The model under review builds one solid part; all positions refer to its coordinate system, in mm. Face numbers are marked on the shaded views. A direction names the side the tool comes from. Give positions to 0.01 mm unless a question says otherwise; leave off trailing zeros. Loops run counter-clockwise (first coordinate to the right, second up) from the corner with the lowest first, then second, coordinate; pieces in that order, holes last. Notation, with made-up numbers: (80, -26.75) - (116, -26.75) arc R10 cw to (116, -21.75) - close; hole circle Ø5 at (58, -20). An arc over 180 degrees is marked (long way). Answer as a JSON object with one key per item and string values.
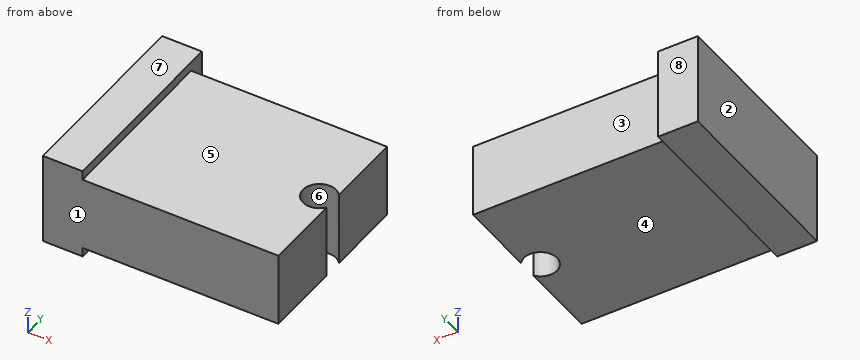
from build123d import *

# Parameters (mm, degrees)
F1_DEPTH = 5.6
F2_D     = 2.5
F2_DEPTH = 12
F3_W     = 13.2
F3_H     = 5.6
F4_DEPTH = 3


with BuildPart() as f1:
    # F0 (on Top) → F1 (new body)
    with BuildSketch(Plane.XY):
        with BuildLine():
            Line((7.4, 6.6), (-7.4, 6.6))
            Line((-7.4, 6.6), (-7.4, 0))
            Line((-7.4, 0), (5.3, 0))
            ThreePointArc((5.3, 0), (6.165479, 1.074709), (7.4, 0.458258))
            Line((7.4, 0.458258), (7.4, 6.6))
        make_face()
        with BuildLine():
            Line((5.3, 0), (-7.4, 0))
            Line((-7.4, 0), (-7.4, -6.6))
            Line((-7.4, -6.6), (7.4, -6.6))
            Line((7.4, -6.6), (7.4, -0.458258))
            ThreePointArc((7.4, -0.458258), (6.165479, -1.074709), (5.3, 0))
        make_face()
        with BuildLine():
            ThreePointArc((7.5, 0), (7.474709, 0.234521), (7.4, 0.458258))
            Line((7.4, 0.458258), (7.4, -0.458258))
            ThreePointArc((7.4, -0.458258), (7.474709, -0.234521), (7.5, 0))
        make_face()
        with BuildLine():
            Line((7.4, -0.458258), (7.4, 0.458258))
            ThreePointArc((7.4, 0.458258), (6.165479, 1.074709), (5.3, 0))
            ThreePointArc((5.3, 0), (6.165479, -1.074709), (7.4, -0.458258))
        make_face()
    extrude(amount=F1_DEPTH)

    # F2
    with Locations(Plane(origin=(0, 0, 0), x_dir=(1, 0, 0), z_dir=(0, 0, -1))):
        with Locations((6.4, 0)):
            Hole(F2_D / 2, depth=F2_DEPTH)

    # F3 (on face) → F4 (join)
    with BuildSketch(Plane(origin=(-7.4, 0, 0), x_dir=(0, -1, 0), z_dir=(-1, 0, 0))):
        Polygon((6.6, 6.3), (-7.9, 6.3), (-7.9, -0.7), (6.6, -0.7), (6.6, 0), (-6.6, 0), (-6.6, 5.6), (6.6, 5.6), align=None)
        with Locations((0, 2.8)):
            Rectangle(F3_W, F3_H)
    extrude(amount=F4_DEPTH)


solid = f1.part
Q1. The part is to be moulded in two halves that separate along Y. For the marked faces 6, 7 and 8, say which applies: +Y half, -Y half, draft (parallel to the pull), parting line (faces both ways), or undercut.
Results:
{"face 6": "undercut", "face 7": "draft", "face 8": "+Y half"}
Q2. Clearance check with flat-ended pins moving along their axes: pin 1 Ø1.5 at (x, z) = (0, 3.5) entering from +Y; pin 2 Ø6 at (x, y) = (-1, -2) entering from -Z. State where each tip first meets the part, or that it passes through.
Results:
{"pin 1": "stops at y = 6.6", "pin 2": "stops at z = 0"}
Q3. Consider section C-C, the plane z = 1. State the section outline as (x, y) points, plus the area to 3 significant figures.
Results:
{"outline": "(-10.4, -6.6) - (7.4, -6.6) - (7.4, -0.75) arc R1.25 cw (long way) to (7.4, 0.75) - (7.4, 6.6) - (-7.4, 6.6) - (-7.4, 7.9) - (-10.4, 7.9) - close", "area": "234 mm^2"}
Q4. Consider section B-B, the plane x = 6.4. State the section outline as (y, z) points.
Results:
{"outline": "(-6.6, 0) - (-1.25, 0) - (-1.25, 5.6) - (-6.6, 5.6) - close; (1.25, 0) - (6.6, 0) - (6.6, 5.6) - (1.25, 5.6) - close"}
Q5. To check wall thickness, follow probe 1 along Y at (x, z) = (6.5, 4); probe 2 along Z at (x, y) = (-1, -4.5); probe 3 along X at (y, z) = (0, 2.45). State the ranges of each line that lie inside material, in increasing order. Write a range as [from, to].
Results:
{"probe 1": "y = [-6.6, -1.25], [1.25, 6.6]", "probe 2": "z = [0, 5.6]", "probe 3": "x = [-10.4, 5.15]"}
Q6. Consider section A-A, the plane y = 1. State the section outline as (x, z) points, plus the area to 3 significant figures.
Results:
{"outline": "(-10.4, -0.7) - (-7.4, -0.7) - (-7.4, 0) - (5.65, 0) - (5.65, 5.6) - (-7.4, 5.6) - (-7.4, 6.3) - (-10.4, 6.3) - close; (7.15, 0) - (7.4, 0) - (7.4, 5.6) - (7.15, 5.6) - close", "area": "95.5 mm^2"}
Q7. Consider section D-D, the plane y = 5.5. State the section outline as (x, z) points, plus the area to 3 significant figures.
Results:
{"outline": "(-10.4, -0.7) - (-7.4, -0.7) - (-7.4, 0) - (7.4, 0) - (7.4, 5.6) - (-7.4, 5.6) - (-7.4, 6.3) - (-10.4, 6.3) - close", "area": "104 mm^2"}
Q8. For the marked faces 1, 2, 3, 4 and 5, list the 3-axis set-ups (+Z, -Z, +X, -X, +Y, -Y) from which the entire face can be reached by the end or side of a thin tool; tool diameter is ignored.
Results:
{"face 1": "+Z, -Z, +X, -X, -Y", "face 2": "+Z, -Z, -X, +Y, -Y", "face 3": "+Z, -Z, +X, +Y", "face 4": "-Z, +X, +Y, -Y", "face 5": "+Z, +X, +Y, -Y"}
